```python
from build123d import *

# Parameters (mm, degrees)
F0_R     = 35.118503
F1_DEPTH = 20.32
F2_R     = 9.100995
F3_DEPTH = 20.32
F4_R     = 7.62


with BuildPart() as f1:
    # F0 (on Front) → F1 (new body)
    with BuildSketch(Plane.XZ):
        Circle(F0_R)
    extrude(amount=F1_DEPTH)

    # F2 (on face) → F3 (cut)
    with BuildSketch(Plane.XZ.offset(20.32)):
        Circle(F2_R)
    extrude(amount=-F3_DEPTH, mode=Mode.SUBTRACT)

    # F4
    f4_edges = [f1.edges().sort_by_distance(p)[0] for p in [
        (-35.118503, 0, 0),
        (-35.118503, -20.32, 0),
        (-9.100995, -20.32, 0),
        (-9.100995, 0, 0),
    ]]
    fillet(f4_edges, radius=F4_R)


solid = f1.part
```
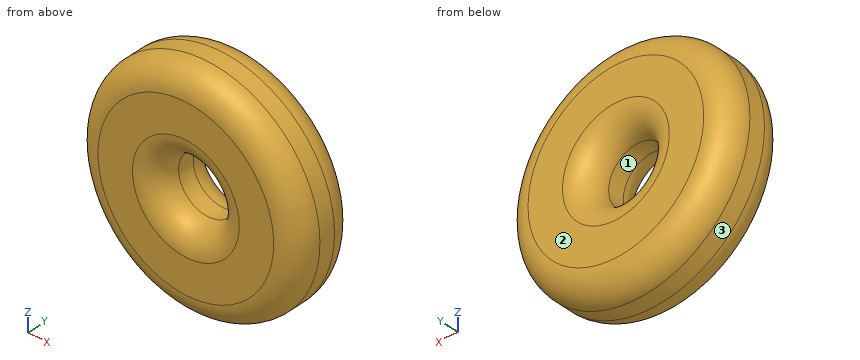
Geometry: final body of the model. Coordinates: model frame, mm. Face numbers are marked on the shaded views. Give positions to 0.01 mm unless a question says otherwise; leave off trailing zeros. Write each loop counter-clockwise with the first axis right and the second up, starting at its lowest first coordinate (ties: lowest second). Pieces come first, ordered by that corner, then holes.
1. Line query: probe 1 along Z at (x, y) = (4.5, -16.25); probe 2 along Z at (x, y) = (-0.5, -5); probe 3 along X at (y, z) = (-3.25, -9.5). Output: solid intervals per line, ascending.
2. Section query B-B, the plane z = 0. Return loops of the section in (x, y), then the cut area to 3 significant figures.
3. Draft query along Z for the marked faces 1, 2 and 3. Return one class per face: released by +Z, released by -Z, zero draft, split by the parting line, or undercut.
4. Section query D-D, the plane y = -2. Return loops of the section in (x, z), then the cut area to 3 significant figures.
5. Pin query (flat end, axial travel): P1, Ø1, axis at x = 25.5, y = -16, coming from the +Z side; P2, Ø1, axis at y = -14, z = -17, coming from the -X side; P3, Ø1.5, axis at x = -13.5, y = -17, coming from the -Z side; P4, Ø16.5, axis at x = 0, z = 0, coming from the +Y side. Return the tip coordinate at first contact, or that it passes through.
6. Section query C-C, the plane y = -9. Return loops of the section in (x, z), then the cut area to 3 significant figures.
7. Section query A-A, the plane x = 0. Return loops of the section in (y, z).
Computed:
1. probe 1: z = -33.94 to -8.91, 8.91 to 33.94
1. probe 2: z = -34.65 to -9.55, 9.55 to 34.65
1. probe 3: x = -32.38 to -4.42, 4.42 to 32.38
2. outline: (-35.12, -12.7) arc R7.62 ccw to (-27.5, -20.32) - (-16.72, -20.32) arc R7.62 ccw to (-9.1, -12.7) - (-9.1, -7.62) arc R7.62 ccw to (-16.72, 0) - (-27.5, 0) arc R7.62 ccw to (-35.12, -7.62) - close; (9.1, -12.7) arc R7.62 ccw to (16.72, -20.32) - (27.5, -20.32) arc R7.62 ccw to (35.12, -12.7) - (35.12, -7.62) arc R7.62 ccw to (27.5, 0) - (16.72, 0) arc R7.62 ccw to (9.1, -7.62) - close
2. area: 958 mm2
3. face 1: undercut
3. face 2: zero draft
3. face 3: split by the parting line
4. outline: circle Ø65.29 at (0, 0); hole circle Ø23.15 at (0, 0)
4. area: 2,930 mm2
5. P1: stops at z = 23.68
5. P2: stops at x = -30.89
5. P3: stops at z = -31.57
5. P4: passes through
6. outline: circle Ø70.24 at (0, 0); hole circle Ø18.2 at (0, 0)
6. area: 3,610 mm2
7. outline: (-20.32, -27.5) arc R7.62 ccw to (-12.7, -35.12) - (-7.62, -35.12) arc R7.62 ccw to (0, -27.5) - (0, -16.72) arc R7.62 ccw to (-7.62, -9.1) - (-12.7, -9.1) arc R7.62 ccw to (-20.32, -16.72) - close; (-20.32, 16.72) arc R7.62 ccw to (-12.7, 9.1) - (-7.62, 9.1) arc R7.62 ccw to (0, 16.72) - (0, 27.5) arc R7.62 ccw to (-7.62, 35.12) - (-12.7, 35.12) arc R7.62 ccw to (-20.32, 27.5) - close
